```python
from build123d import *

# Parameters (mm, degrees)
EXTRUDE_1_DEPTH     = 30
CUT_EXTRUDE_1_DEPTH = 69.738635424
EXTRUDE_2_DEPTH     = 30
SKETCH_4_R          = 30
EXTRUDE_3_DEPTH     = 13
EXTRUDE_4_DEPTH     = 3
CUT_EXTRUDE_2_REACH = 102.632
SKETCH_5_R          = 7
RIB_1_REACH         = 102.196
SKETCH_6_WALL_W     = 230.660820914
SKETCH_6_WALL_H     = 10


with BuildPart() as part:
    # 草图1 → 凸台-拉伸1 (new, symmetric)
    with BuildSketch(Plane.XY):
        Polygon((-25, 0), (-25, -3), (-60, -3), (-60, 12), (60, 12), (60, -3), (25, -3), (25, 0), align=None)
    extrude(amount=EXTRUDE_1_DEPTH, both=True)

    # 草图2 → 切除-拉伸1 (cut, through all)
    with BuildSketch(Plane(origin=(0, 12, 0), x_dir=(1, 0, 0), z_dir=(0, 1, 0))):
        with BuildLine():
            Line((75, -7), (45, -7))
            ThreePointArc((45, -7), (38, 0), (45, 7))
            Line((45, 7), (75, 7))
            ThreePointArc((75, 7), (82, 0), (75, -7))
        make_face()
        with BuildLine():
            Line((-75, -7), (-45, -7))
            ThreePointArc((-45, -7), (-38, 0), (-45, 7))
            Line((-45, 7), (-75, 7))
            ThreePointArc((-75, 7), (-82, 0), (-75, -7))
        make_face()
    extrude(amount=-CUT_EXTRUDE_1_DEPTH, mode=Mode.SUBTRACT)

    # 草图3 → 凸台-拉伸2 (add, symmetric)
    with BuildSketch(Plane.XY):
        Polygon((-10, 12), (2, 12), (2, 32), (-19.213203436, 53.213203436), (-28.405591591, 44.02081528), (-10, 25.615223689), align=None)
    extrude(amount=EXTRUDE_2_DEPTH, both=True)

    # 草图4 → 凸台-拉伸3 (add)
    with BuildSketch(Plane(origin=(17, 17, 0), x_dir=(0, 0, -1), z_dir=(0.7071067811865483, 0.7071067811865468, 0))):
        with Locations((0, 51.213203436)):
            Circle(SKETCH_4_R)
    extrude(amount=-EXTRUDE_3_DEPTH)

    # 草图4<3> → 凸台-拉伸4 (add)
    with BuildSketch(Plane(origin=(17, 17, 0), x_dir=(0, 0, -1), z_dir=(0.7071067811865483, 0.7071067811865468, 0))):
        with BuildLine():
            Line((7, 51.213203436), (20, 51.213203436))
            ThreePointArc((20, 51.213203436), (0, 71.213203436), (-20, 51.213203436))
            Line((-20, 51.213203436), (-7, 51.213203436))
            ThreePointArc((-7, 51.213203436), (0, 58.213203436), (7, 51.213203436))
        make_face()
        with BuildLine():
            ThreePointArc((-20, 51.213203436), (0, 31.213203436), (20, 51.213203436))
            Line((20, 51.213203436), (7, 51.213203436))
            ThreePointArc((7, 51.213203436), (0, 44.213203436), (-7, 51.213203436))
            Line((-7, 51.213203436), (-20, 51.213203436))
        make_face()
    extrude(amount=EXTRUDE_4_DEPTH)

    # 草图5 → 切除-拉伸2 (cut, up to next)
    with BuildSketch(Plane(origin=(17, 17, 0), x_dir=(0, 0, -1), z_dir=(0.7071067811865483, 0.7071067811865468, 0)), mode=Mode.PRIVATE) as cut_extrude_2_sk1:
        with Locations(Location((0, 51.213203436, 0), (0, 0, 90))):
            Circle(SKETCH_5_R)
    cut_extrude_2_tool1 = extrude(cut_extrude_2_sk1.sketch, amount=-CUT_EXTRUDE_2_REACH, mode=Mode.PRIVATE) & part.part
    add(cut_extrude_2_tool1.solids().sort_by_distance((-19.213203, 53.213203, 0))[0], mode=Mode.SUBTRACT)

    # 草图6 wall → 筋1 (add, up to next)
    with BuildSketch(Plane(origin=(-27.932923579, 24.240535423, 0), x_dir=(-0.5, -0.866025403784, 0), z_dir=(0.866025403784, -0.5, 0)), mode=Mode.PRIVATE) as rib_1_sk1:
        Rectangle(SKETCH_6_WALL_W, SKETCH_6_WALL_H)
    rib_1_tool1 = extrude(rib_1_sk1.sketch, amount=RIB_1_REACH, mode=Mode.PRIVATE) - part.part
    add(rib_1_tool1.solids().sort_by_distance((-27.932923579, 24.240535423, 0))[0])


solid = part.part
```
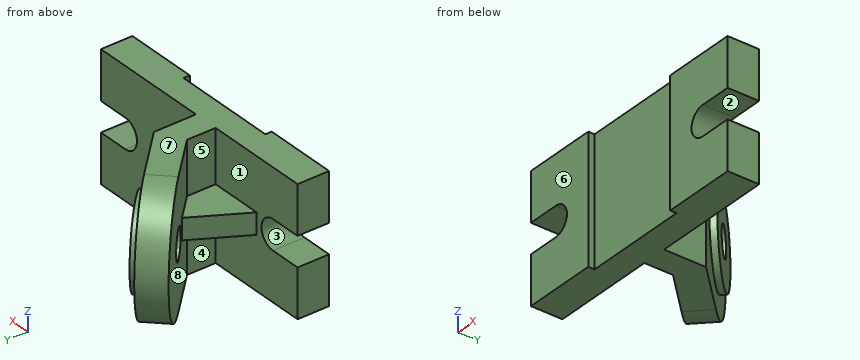
Geometry check sheet. Reference: the model listing, model coordinates, mm. Face numbers are marked on the shaded views. A direction names the side the tool comes from. Give positions to 0.01 mm unless a question says otherwise; leave off trailing zeros. Order: outer loops, then holes, each group sorted by start corner. A loop starts at its lowest first (then second) coordinate and runs counter-clockwise, first axis right, second up. Notation, with made-up numbers: (-32, 16) - (16, 16) arc R9 ccw to (16, 20) - close; hole circle Ø7 at (45, 52.5). An arc over 180 degrees is marked (long way). Write item = value, one per line. Start each with the question number.
1) Section check A-A (x = 48). Enter the section's corners in (y, z).
2) Section check D-D (x = 7). Enter the section's corners in (y, z), then the cut area to 3 significant figures.
3) Draft check along Y on the marked faces 6, 7 and 8. Enter one of: released by +Y, released by -Y, zero draft, split by the parting line, or undercut.
4) Section check C-C (z = 18.5). Enter the section's corners in (x, y).
5) Section check B-B (z = 0). Enter the section's corners in (x, y).
6) Gauge pin test, flat ends, axial feed: pin 1 Ø22 at (y, z) = (23.5, 8.5) entering from +X; pin 2 Ø7.5 at (x, y) = (-27.5, 28) entering from -Z; pin 3 Ø6 at (x, z) = (18, -23) entering from +Y. Record the tip position at first contact, or that the pin passes through.
7) Access from +Z, -Z, +X, -X, +Y, -Y to the whole of each face (thin tool, end or side, straight path). Record for the marked faces 1, 2, 3, 4 and 5.
8) Scan lines: L1, parallel to Z at x = 45, y = 10; L2, parallel to Y at x = 31, z = 8; L3, parallel to Y at x = -25.5, z = -3.5. Record each from-to range of solid material in increasing order.
Geometry check:
q1.outline = (-3, -30) - (12, -30) - (12, -7) - (-3, -7) - close; (-3, 7) - (12, 7) - (12, 30) - (-3, 30) - close
q2.outline = (0, -30) - (12, -30) - (12, 30) - (0, 30) - close
q2.area = 720 mm2
q3.face_6 = released by -Y
q3.face_7 = zero draft
q3.face_8 = undercut
q4.outline = (-60, -3) - (-25, -3) - (-25, 0) - (25, 0) - (25, -3) - (60, -3) - (60, 12) - (2, 12) - (2, 32) - (-13.84, 47.84) - (-11.72, 49.96) - (-22.47, 60.71) - (-24.59, 58.59) - (-35.91, 69.91) - (-45.11, 60.72) - (-10, 25.62) - (-10, 12) - (-60, 12) - close
q5.outline = (-49.62, 65.23) - (-33.36, 48.97) - (-22.04, 60.28) - (-31.23, 69.48) - (-33.36, 67.36) - (-40.43, 74.43) - close; (-38, -3) - (-25, -3) - (-25, 0) - (25, 0) - (25, -3) - (38, -3) - (38, 12) - (2, 12) - (2, 32) - (-5.07, 39.07) - (-2.95, 41.19) - (-12.14, 50.38) - (-23.46, 39.07) - (-20.87, 36.48) - (-35, 12) - (-38, 12) - close
q6.pin_1 = 2
q6.pin_2 = -5
q6.pin_3 = 12
q7.face_1 = -X
q7.face_2 = +X, +Y, -Y
q7.face_3 = -X, -Y
q7.face_4 = -Z, -X
q7.face_5 = +Z, -X
q8.L1 = -30 to -7, 7 to 30
q8.L2 = -3 to 12
q8.L3 = -3 to 28.45, 55.5 to 63.74
